The drawing under review shows one solid part. Ordinate dimensions are in mm from its lowest x, y, z. A direction names the side the tool comes from. Give positions to 0.01 mm unless a question says otherwise; leave off trailing zeros. Write each loop counter-clockwise with the first axis right and the second up, starting at its lowest first coordinate (ties: lowest second). Pieces come first, ordered by that corner, then holes. Notation, with made-up numbers: (51.5, 23) -> (68.5, 23) arc R34 ccw to (68.5, 55) -> close; hole circle Ø4 at (-35.5, 18). An arc over 180 degrees is marked (long way). Put each result on its own line as item: value. Start each with the question number.
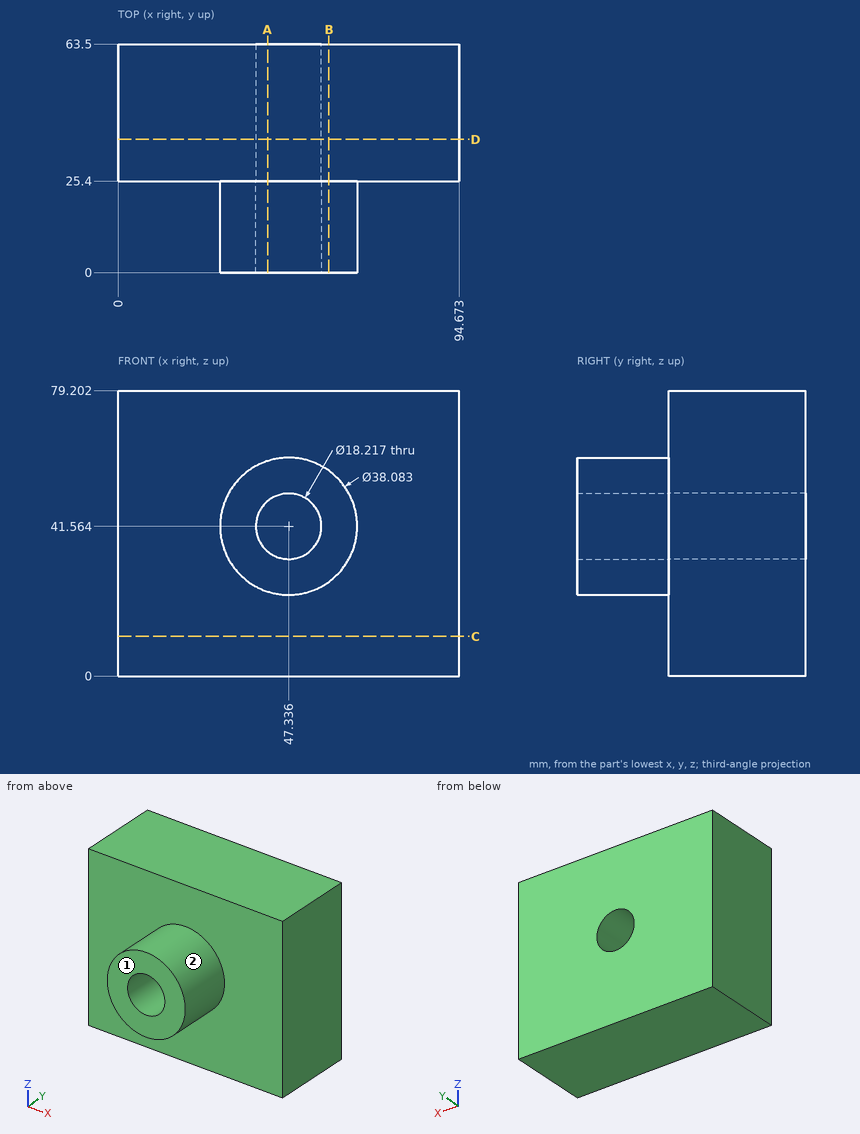
Q1. Take a section at D-D on y = 37. Give the boundary of the cut face in (x, z) (1 decimal).
Q2. Machinability: for the marked faces 1 and 2, which of the approach directions +Z, -Z, +X, -X, +Y, -Y give a long, thin tool a straight path to every point of the face, cutting with its end or side? Answer none if there is none.
Q3. Take a section at C-C on z = 11. Give the boundary of the cut face in (x, y), then the cut area to 3 significant figures.
Q4. Take a section at B-B on x = 58.5. Give the boundary of the cut face in (y, z), then the cut area to 3 significant figures.
Q5. For pin 1 (2 mm diameter, centred on x = 40, y = 13, fed in from -Z); pin 2 (6 mm diameter, centred on x = 58, z = 62, fed in from -Y); pin 3 (2 mm diameter, centred on x = 29.5, y = 14, fed in from -Z), all flat-tipped, find the tip position at first contact; note any pin that passes through.
Q6. To check wall thickness, follow probe 1 along Y at (x, z) = (84, 46.5); probe 2 along Z at (x, y) = (51, 48.5) (1 decimal); probe 3 along X at (y, z) = (17.5, 45) (1 decimal). State the ranges of each line that lie inside material, in increasing order. Write a range as from..to.
Q7. Take a section at A-A on x = 41.5. Give the boundary of the cut face in (y, z).
Result:
1. outline: (0, 0) -> (94.7, 0) -> (94.7, 79.2) -> (0, 79.2) -> close; hole circle Ø18.2 at (47.3, 41.6)
2. face 1: +Z, -Z, +X, -X, -Y
2. face 2: -Y
3. outline: (0, 25.4) -> (94.67, 25.4) -> (94.67, 63.5) -> (0, 63.5) -> close
3. area: 3,610 mm^2
4. outline: (0, 26.14) -> (25.4, 26.14) -> (25.4, 0) -> (63.5, 0) -> (63.5, 79.2) -> (25.4, 79.2) -> (25.4, 56.99) -> (0, 56.99) -> close
4. area: 3,800 mm^2
5. pin 1: stops at z = 23.61
5. pin 2: stops at y = 25.4
5. pin 3: stops at z = 32.67
6. probe 1: y = 25.4..63.5
6. probe 2: z = 0..33.2, 49.9..79.2
6. probe 3: x = 28.6..38.9, 55.8..66.1
7. outline: (0, 23.44) -> (25.4, 23.44) -> (25.4, 0) -> (63.5, 0) -> (63.5, 34.57) -> (0, 34.57) -> close; (0, 48.56) -> (63.5, 48.56) -> (63.5, 79.2) -> (25.4, 79.2) -> (25.4, 59.69) -> (0, 59.69) -> close
